Solid Edge part; units mm, degrees
sketch "Sketch1" plane through (0, 0, 0) normal (0, -1, 0) x (1, 0, 0)
  line L0 (-13.1317, 37) -> (0, 37)
  line L1 (13.1317, 37) -> (0, 37)
  line L2 (26.2132, 0) -> (13.1317, 37)
  line L3 (0, 0) -> (26.2132, 0)
  line L4 (0, 0) -> (-26.2132, 0)
  line L5 (-26.2132, 0) -> (-13.1317, 37)
  circle A0 centre (-5, 30) radius 2.5
  circle A1 centre (5, 30) radius 2.5
  circle A2 centre (-5, 15) radius 7.5
extrude "Protrusion1" add sketch "Sketch1" along normal mid plane 20
Can you work these out from the model? Positions are in its coordinate system, mm. Coordinates: 2 decimals unless noted, no trailing zeros. Loops run counter-clockwise (first coordinate to the right, second up) from the corner with the lowest first, then second, coordinate; pieces in that order, holes last.
Item 1: Suppose I cut it at C-C (x = 5). Please give me the cut outline in (y, z).
Answers below:
outline: (-10, 0) - (10, 0) - (10, 27.5) - (-10, 27.5) - close; (-10, 32.5) - (10, 32.5) - (10, 37) - (-10, 37) - close
Item 2: I'm going to push flat-ended pins straight in: pin 1 (8 mm diameter, centred on y = 0, z = 28.5, fed in from +X); pin 2 (4.5 mm diameter, centred on x = 5, z = 30, fed in from -Y); pin 3 (4 mm diameter, centred on y = -3, z = 5.5, fed in from +X); pin 4 (10 mm diameter, centred on y = 4, z = 10.5, fed in from +X). Where does each tip first touch, or does it pass through?
Answers below:
pin 1: stops at x = 17.55
pin 2: passes through
pin 3: stops at x = 24.98
pin 4: stops at x = 24.27
Item 3: Suppose I cut it at A-A (x = -5). Please give me the cut outline in (y, z), then the cut area to 3 significant figures.
Answers below:
outline: (-10, 0) - (10, 0) - (10, 7.5) - (-10, 7.5) - close; (-10, 22.5) - (10, 22.5) - (10, 27.5) - (-10, 27.5) - close; (-10, 32.5) - (10, 32.5) - (10, 37) - (-10, 37) - close
area: 340 mm2
Item 4: Please list where these lines run through material, in increasing order: L1, parallel to Z at x = 5, y = 6; L2, parallel to Z at x = -5, y = -3.25; L3, parallel to X at y = -0.5, z = 17.
Answers below:
L1: z = 0 to 27.5, 32.5 to 37
L2: z = 0 to 7.5, 22.5 to 27.5, 32.5 to 37
L3: x = -20.2 to -12.23, 2.23 to 20.2
Item 5: Suppose I cut it at D-D (z = 15). Please give me the cut outline in (x, y), then the cut area to 3 significant figures.
Answers below:
outline: (-20.91, -10) - (-12.5, -10) - (-12.5, 10) - (-20.91, 10) - close; (2.5, -10) - (20.91, -10) - (20.91, 10) - (2.5, 10) - close
area: 536 mm2
Item 6: If we mould it in two halves opening along X, with no side actions, what happens to faces 1 (the face through (-19.764, 0.14, 18.241)), 2 (the face through (-3.66, 0.14, 27.89)), 3 (the face through (6, -10, 14))? For each: released by +X, released by -X, zero draft, split by the parting line, or undercut.
Answers below:
face 1: released by -X
face 2: undercut
face 3: zero draft
Item 7: Suppose I cut it at B-B (y = 7). Please give me the cut outline in (x, z).
Answers below:
outline: (-26.21, 0) - (26.21, 0) - (13.13, 37) - (-13.13, 37) - close; hole circle Ø15 at (-5, 15); hole circle Ø5 at (-5, 30); hole circle Ø5 at (5, 30)
